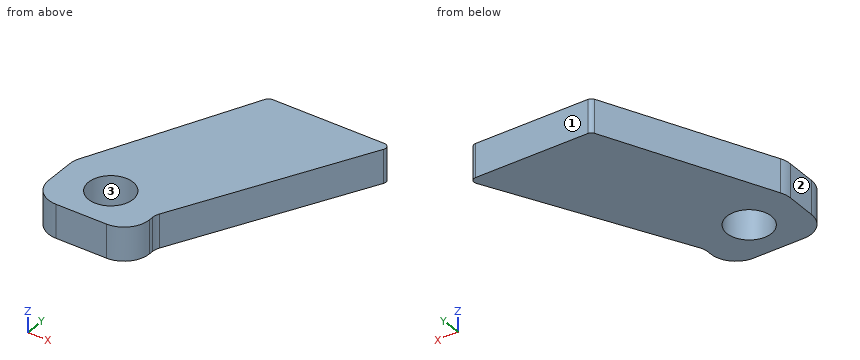
```python
from build123d import *

# Parameters (mm, degrees)
SKETCH1_R          = 13.25
BASE_EXTRUDE_DEPTH = 20


with BuildPart() as part:
    # Sketch1 → Base-Extrude (new body)
    with BuildSketch(Plane.XY):
        with BuildLine():
            Line((30, -7.446984432), (30, -10))
            ThreePointArc((30, -10), (25.606601718, -20.606601718), (15, -25))
            Line((15, -25), (-15, -25))
            ThreePointArc((-15, -25), (-25.606601718, -20.606601718), (-30, -10))
            Line((-30, -10), (-30, 7.67458006))
            ThreePointArc((-30, 7.67458006), (-29.644440107, 10.921174269), (-28.594616806, 14.013853986))
            Line((-28.594616806, 14.013853986), (15.589899408, 108.767854785))
            ThreePointArc((15.589899408, 108.767854785), (16.696923944, 110.030174337), (18.308822769, 110.5))
            Line((18.308822769, 110.5), (85.181647346, 110.5))
            ThreePointArc((85.181647346, 110.5), (87.746382958, 109.056319774), (87.842679846, 106.11475416))
            Line((87.842679846, 106.11475416), (31.129891668, -2.8294983))
            ThreePointArc((31.129891668, -2.8294983), (30.286579302, -5.070125509), (30, -7.446984432))
        make_face()
        Circle(SKETCH1_R, mode=Mode.SUBTRACT)
    extrude(amount=BASE_EXTRUDE_DEPTH)


solid = part.part
```
The model under review builds one solid part; all positions refer to its coordinate system, in mm. Face numbers are marked on the shaded views. Give positions to 0.01 mm unless a question says otherwise; leave off trailing zeros. Loops run counter-clockwise (first coordinate to the right, second up) from the corner with the lowest first, then second, coordinate; pieces in that order, holes last. Notation, with made-up numbers: (15.5, 62.25) - (73.5, 62.25) arc R25 cw to (73.5, 93.25) - close; hole circle Ø6 at (71, 70.25). An arc over 180 degrees is marked (long way). Answer as a JSON object with one key per item and string values.
Q1. Insertion check: pin 1 (3 mm diameter, centred on x = 70, z = 6, fed in from -Y); pin 2 (1.5 mm diameter, centred on x = 34.5, z = 16.5, fed in from -Y); pin 3 (0.8 mm diameter, centred on y = -9, z = 10, fed in from +X). Each pin has a flat end and moves straight along its axis. Give the tip position at first contact, or say it passes through.
Worked out:
{"pin 1": "stops at y = 68.96", "pin 2": "stops at y = 2.2", "pin 3": "stops at x = 30"}
Q2. Mouldability with a two-part tool opening along Y and no side actions: class the marked faces 1, 2 and 3 as +Y half, -Y half, draft (parallel to the pull), parting line (faces both ways), or undercut.
Worked out:
{"face 1": "+Y half", "face 2": "draft", "face 3": "undercut"}
Q3. Add section B-B on x = 0. State the section outline as (y, z) points, plus the area to 3 significant figures.
Worked out:
{"outline": "(-25, 0) - (-13.25, 0) - (-13.25, 20) - (-25, 20) - close; (13.25, 0) - (75.34, 0) - (75.34, 20) - (13.25, 20) - close", "area": "1,480 mm^2"}
Q4. To check wall thickness, follow line 1 along Y through (x, z) = (0, 8.5); line 2 along X through (y, z) = (4.5, 16); line 3 along Y through (x, z) = (-3, 12.25). State the ranges of each line that lie inside material, in increasing order.
Worked out:
{"line 1": "y = -25 to -13.25, 13.25 to 75.34", "line 2": "x = -30 to -12.46, 12.46 to 34.95", "line 3": "y = -25 to -12.91, 12.91 to 68.9"}
Q5. Add section D-D on x = 54.5. State the section outline as (y, z) points.
Worked out:
{"outline": "(42.06, 0) - (110.5, 0) - (110.5, 20) - (42.06, 20) - close"}
Q6. Add section A-A on z = 14. State the section outline as (x, y) points, plus the area to 3 significant figures.
Worked out:
{"outline": "(-30, -10) arc R15 ccw to (-15, -25) - (15, -25) arc R15 ccw to (30, -10) - (30, -7.45) arc R10 cw to (31.13, -2.83) - (87.84, 106.11) arc R3 ccw to (85.18, 110.5) - (18.31, 110.5) arc R3 ccw to (15.59, 108.77) - (-28.59, 14.01) arc R15 ccw to (-30, 7.67) - close; hole circle Ø26.5 at (0, 0)", "area": "8,640 mm^2"}
Q7. Add section C-C on y = 0. State the section outline as (x, z) points, plus the area to 3 significant figures.
Worked out:
{"outline": "(-30, 0) - (-13.25, 0) - (-13.25, 20) - (-30, 20) - close; (13.25, 0) - (32.6, 0) - (32.6, 20) - (13.25, 20) - close", "area": "722 mm^2"}
